Geometry: final body of the model. Coordinates: model frame, mm. Coordinates: 2 decimals unless noted, no trailing zeros. Order: outer loops, then holes, each group sorted by start corner. A loop starts at its lowest first (then second) coordinate and runs counter-clockwise, first axis right, second up. Notation, with made-up numbers: M 64.5,77 L 121.5,77 A18 cw 121.5,89 Z; hole C 75,-7.75 d3. An arc over 180 degrees is marked long. Use CSV: the item, a comma, the result in double quotes. Start each with the question number.
1. Material intervals for line 1 (X direction, y = 26, z = 23); line 2 (Z direction, x = 346, y = 27); line 3 (Y direction, x = 312, z = 16.75), sorted ascending.
2. Section query B-B on y = 28.5. Return the cut outline in (x, z).
3. Section query A-A on z = 23. Return the cut outline in (x, y), and give its area (3 significant figures).
4. Section query C-C on x = 522.5. Return the cut outline in (y, z), and give its area (3 significant figures).
5. First-contact query: P1, Ø6, axis at x = 139, y = 25.5, coming from the +Z side; P2, Ø16.5, axis at x = 298, z = 25, coming from the +Y side; P3, Ø16.5, axis at x = 662, z = 22.5, coming from the +Y side. Flat tips, straight axial feed; report the tip coordinate or a pass-through.
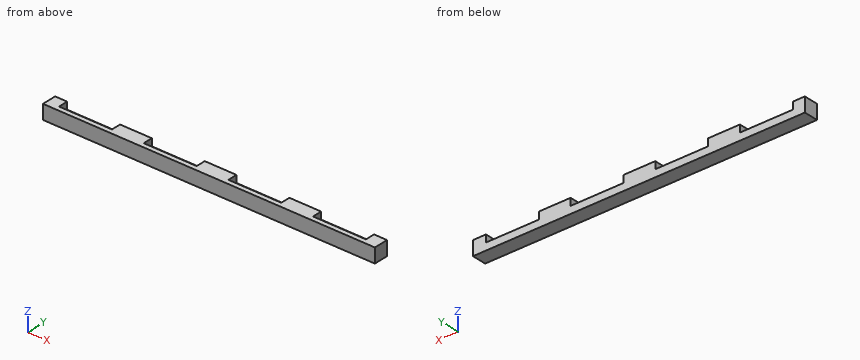
from build123d import *

# Parameters (mm, degrees)
SKETCH_1_W             = 690
SKETCH_1_H             = 30
EXTRUDE_1_DEPTH        = 30
SKETCH_2_W             = 110
SKETCH_2_H             = 15
CUT_EXTRUDE_1_DEPTH    = 20
PATTERN_LINEAR_1_COUNT = 4
PATTERN_LINEAR_1_PITCH = 176


with BuildPart() as part:
    # Эскиз1 → Бобышка-Вытянуть1 (new body)
    with BuildSketch(Plane.XY):
        with Locations((389.050320868, 22.631091658)):
            Rectangle(SKETCH_1_W, SKETCH_1_H)
    extrude(amount=EXTRUDE_1_DEPTH)

    # Эскиз2 → Вырез-Вытянуть1 (cut)
    with BuildSketch(Plane(origin=(0, 37.631091658, 0), x_dir=(1, 0, 0), z_dir=(0, 1, 0))):
        with Locations((124.050320868, -22.5)):
            Rectangle(SKETCH_2_W, SKETCH_2_H)
    cut_extrude_1 = extrude(amount=-CUT_EXTRUDE_1_DEPTH, mode=Mode.SUBTRACT)

    # Линейный массив1: Вырез-Вытянуть1 ×4
    with Locations(*[(i * PATTERN_LINEAR_1_PITCH, 0, 0) for i in range(1, PATTERN_LINEAR_1_COUNT)]):
        add(cut_extrude_1, mode=Mode.SUBTRACT)


solid = part.part
Results list:
1,line 1,"x = 44.05 to 69.05, 179.05 to 245.05, 355.05 to 421.05, 531.05 to 597.05, 707.05 to 734.05"
1,line 2,"z = 0 to 15"
1,line 3,"y = 7.63 to 17.63"
2,outline,"M 44.05,0 L 734.05,0 L 734.05,30 L 707.05,30 L 707.05,15 L 597.05,15 L 597.05,30 L 531.05,30 L 531.05,15 L 421.05,15 L 421.05,30 L 355.05,30 L 355.05,15 L 245.05,15 L 245.05,30 L 179.05,30 L 179.05,15 L 69.05,15 L 69.05,30 L 44.05,30 Z"
3,outline,"M 44.05,7.63 L 734.05,7.63 L 734.05,37.63 L 707.05,37.63 L 707.05,17.63 L 597.05,17.63 L 597.05,37.63 L 531.05,37.63 L 531.05,17.63 L 421.05,17.63 L 421.05,37.63 L 355.05,37.63 L 355.05,17.63 L 245.05,17.63 L 245.05,37.63 L 179.05,37.63 L 179.05,17.63 L 69.05,17.63 L 69.05,37.63 L 44.05,37.63 Z"
3,area,"11,900 mm²"
4,outline,"M 7.63,0 L 37.63,0 L 37.63,15 L 17.63,15 L 17.63,30 L 7.63,30 Z"
4,area,"600 mm²"
5,P1,"stops at z = 15"
5,P2,"stops at y = 17.63"
5,P3,"stops at y = 37.63"
